Input: dimensioned drawing with shaded views. Units: mm. Origin: part minimum x, y, z. Coordinates: 2 decimals unless noted, no trailing zeros. Order: outer loops, then holes, each group sorted by start corner. A loop starts at its lowest first (then second) coordinate and runs counter-clockwise, first axis right, second up. Notation, with made-up numbers: M -28.5,41 L 13.5,41 A28 ccw 13.5,79 Z; hole C 7.5,-12.75 d8. An arc over 180 degrees is marked long. Write item = value, one per line.
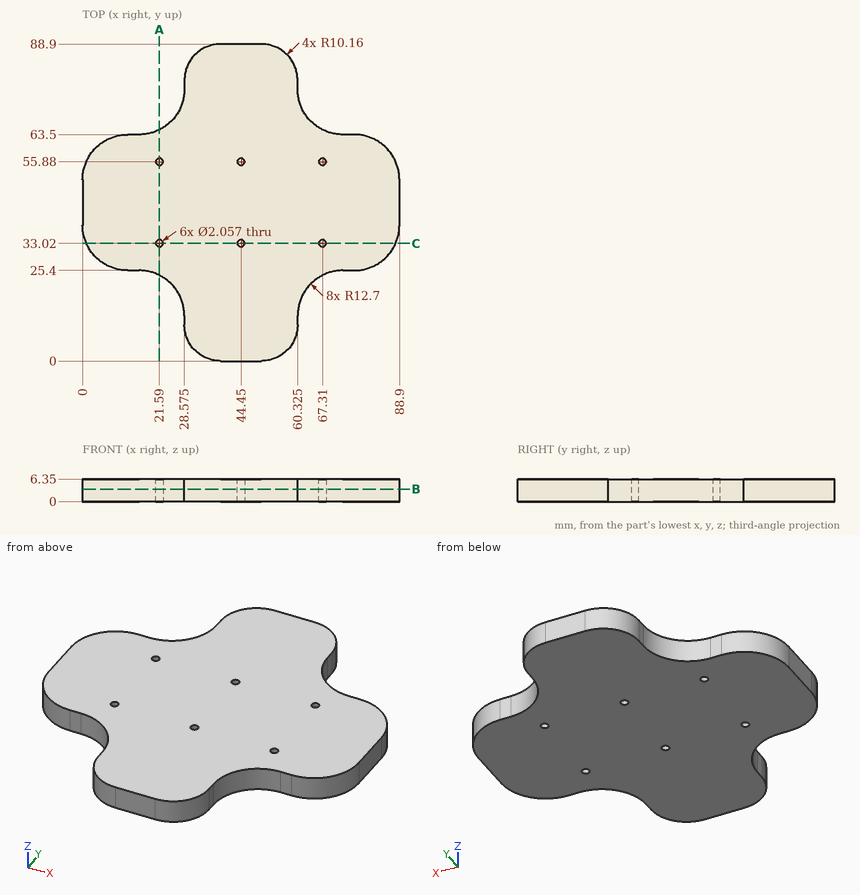
1) Pin query (flat end, axial travel): pin 1 (1.6 mm diameter, centred on x = 21.59, y = 55.88, fed in from +Z); pin 2 (1.3 mm diameter, centred on y = 78, z = 2.5, fed in from -X) (3 decimals); pin 3 (3.5 mm diameter, centred on x = 14, z = 4.5, fed in from +Y); pin 4 (0.8 mm diameter, centred on y = 77, z = 2, fed in from +X) (3 decimals). Return the tip coordinate at first contact, or that it passes through.
Numbers:
pin_1 = through
pin_2 = 28.575
pin_3 = 63.5
pin_4 = 60.325
2) Section A-A, the plane x = 21.59. Return loops of the section in (y, z).
Numbers:
outline = M 24.04,0 L 31.99,0 L 31.99,6.35 L 24.04,6.35 Z; M 34.05,0 L 54.85,0 L 54.85,6.35 L 34.05,6.35 Z; M 56.91,0 L 64.86,0 L 64.86,6.35 L 56.91,6.35 Z
3) Line query: L1, parallel to Y at x = 44.45, z = 3; L2, parallel to Y at x = 67.31, z = 4; L3, parallel to X at y = 33, z = 3. Output: solid intervals per line, ascending.
Numbers:
L1 = 0 to 31.99, 34.05 to 54.85, 56.91 to 88.9
L2 = 24.04 to 31.99, 34.05 to 54.85, 56.91 to 64.86
L3 = 1.07 to 20.56, 22.62 to 43.42, 45.48 to 66.28, 68.34 to 87.83
4) Section B-B, the plane z = 3.5. Give the number of separate pieces and of enclosed holes in the cut face, and give its area (3 significant figures).
Numbers:
separate_pieces = 1
enclosed_holes = 6
area = 4,890 mm²
5) Section C-C, the plane y = 33.02. Return loops of the section in (x, z), and give its area (3 significant figures).
Numbers:
outline = M 1.06,0 L 20.56,0 L 20.56,6.35 L 1.06,6.35 Z; M 22.62,0 L 43.42,0 L 43.42,6.35 L 22.62,6.35 Z; M 45.48,0 L 66.28,0 L 66.28,6.35 L 45.48,6.35 Z; M 68.34,0 L 87.84,0 L 87.84,6.35 L 68.34,6.35 Z
area = 512 mm²
